Part print with two shaded views. Sizes in mm from the minimum x, y, z corner. A direction names the side the tool comes from. Coordinates: 2 decimals unless noted, no trailing zeros. Loops run counter-clockwise (first coordinate to the right, second up) from the corner with the lowest first, then second, coordinate; pieces in that order, holes last.
(1) Two-plate mould, pull along Z, no slides. Class the marked faces 3, 4 and 5: pulls with the +Z half, pulls with the -Z half, needs draft (parallel to the pull), parting line crosses it, or undercut.
(2) Slice it at C-C (x = 24.5). Give the cut face in (y, z).
(3) Tool access for the marked faces 1 and 2: list every direction of +Z, -Z, +X, -X, +Y, -Y with a clear straight run to the whole face (end or side of a thin tool).
(4) Flat gauge pins, fed straight in: P1, Ø25, axis at y = 62.5, z = 106.95, coming from the -X side; P2, Ø2, axis at x = 25, z = 51.5, coming from the -Y side; P3, Ø1, axis at x = 34, y = 77.5, coming from the +Z side (1 decimal). Where does each tip first touch, or does it go through?
(5) Slice it at B-B (z = 108). Give the cut face in (x, y).
(6) Slice it at A-A (z = 62.5). Give the number of separate pieces and of enclosed holes in the cut face, and give its area (3 significant figures).
(7) Slice it at D-D (y = 102.5). Give the cut face in (x, z), and give its area (3 significant figures).
(8) Wall check: L1, parallel to X at y = 7.5, z = 78; L2, parallel to Z at x = 41, y = 69 (1 decimal); L3, parallel to Z at x = 6.5, y = 106.95 (1 decimal). Give the ranges that are in metal, low to high.
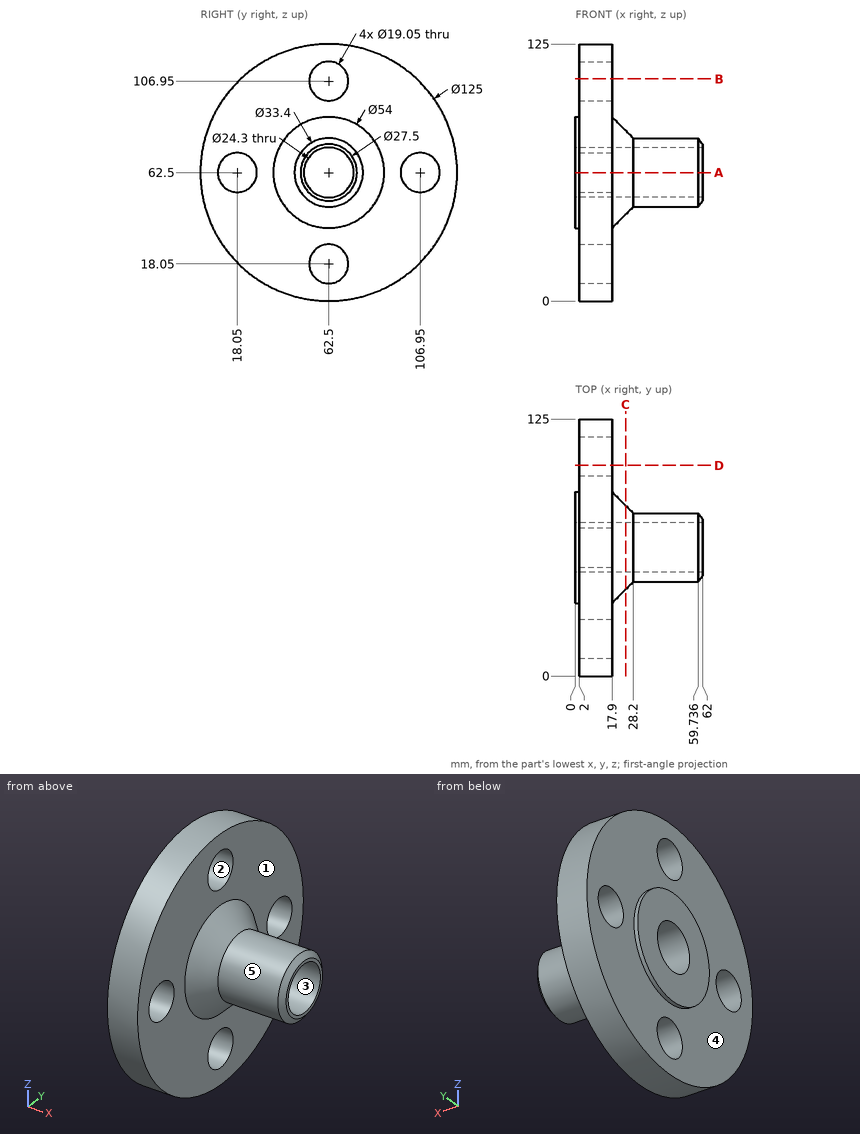
Response values:
1. face 3: undercut
1. face 4: needs draft
1. face 5: parting line crosses it
2. outline: circle Ø40.8 at (62.5, 62.5); hole circle Ø24.3 at (62.5, 62.5)
3. face 1: +X
3. face 2: +X, -X
4. P1: stops at x = 2
4. P2: stops at y = 44.58
4. P3: stops at z = 70.8
5. outline: (2, 19.65) - (17.9, 19.65) - (17.9, 53.03) - (2, 53.03) - close; (2, 71.97) - (17.9, 71.97) - (17.9, 105.35) - (2, 105.35) - close
6. separate pieces: 4
6. enclosed holes: 0
6. area: 1,560 mm2
7. outline: (2, 14.48) - (17.9, 14.48) - (17.9, 54.08) - (2, 54.08) - close; (2, 70.92) - (17.9, 70.92) - (17.9, 110.52) - (2, 110.52) - close
7. area: 1,260 mm2
8. L1: x = 2 to 17.9
8. L2: z = 47.1 to 52.2, 72.8 to 77.9
8. L3: z = 18.6 to 53, 72 to 106.4
